```python
from build123d import *

# Parameters (mm, degrees)
SKETCH1_W                = 63.5
SKETCH1_H                = 50.8
BOSS_EXTRUDE1_DEPTH      = 6.35
F_10_32_THREADED_D       = 4.826
F_10_32_THREADED_FRONT_D = 4.826
F_6_32_THREADED_FRONT_D  = 3.5052


with BuildPart() as part:
    # Sketch1 → Boss-Extrude1 (new, symmetric)
    with BuildSketch(Plane.XY):
        with Locations((-31.75, 25.4)):
            Rectangle(SKETCH1_W, SKETCH1_H)
    extrude(amount=BOSS_EXTRUDE1_DEPTH, both=True)

    # #10-32 Threaded (through all)
    with Locations(Plane(origin=(0, 0, 0), x_dir=(0, 0, -1), z_dir=(1, 0, 0))):
        with Locations((0, 44.45), (0, 25.4), (0, 6.35)):
            Hole(F_10_32_THREADED_D / 2)

    # #10-32 Threaded Front (through all)
    with Locations(Plane.XY.offset(6.35)):
        with Locations((-50.8, 38.1), (-25.4, 38.1), (-50.8, 12.7), (-25.4, 12.7)):
            Hole(F_10_32_THREADED_FRONT_D / 2)

    # #6-32 Threaded Front (through all)
    with Locations(Plane.XY.offset(6.35)):
        with Locations((-34.925, 34.925), (-15.875, 34.925), (-15.875, 15.875), (-34.925, 15.875)):
            Hole(F_6_32_THREADED_FRONT_D / 2)


solid = part.part
```
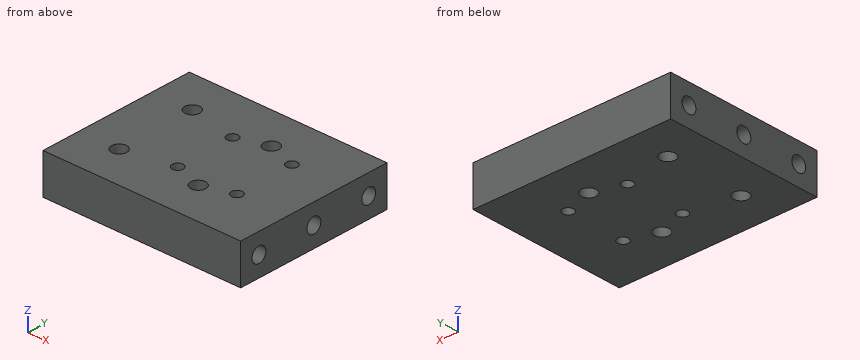
Build history of the part. All positions in model axes, mm. Round coordinates to 2 decimals unless told otherwise and drop trailing zeros. Write each loop counter-clockwise with the first axis right and the second up, starting at its lowest first coordinate (ties: lowest second). Pieces come first, ordered by that corner, then holes.
1) Band-saw the part on D-D, the plane z = -0.5. Give the number of separate pieces and of enclosed holes in the cut face, and give its area (3 significant figures).
2) Band-saw the part on B-B, the plane y = 12.7. List the corners of the cut face in (x, z), and give its area (3 significant figures).
3) Band-saw the part on C-C, the plane y = 6.35. List the corners of the cut face in (x, z), and give its area (3 significant figures).
4) Drill centre lines: probe 1 along Y at (x, z) = (-50.8, -0.25); probe 2 along Y at (x, z) = (-37.5, 0); probe 3 along Z at (x, y) = (-34, 44.5). Where is each one in solid material? Low to high.
5) Band-saw the part on A-A, the plane x = -25.4. List the corners of the cut face in (y, z).
Ans:
1. separate pieces: 4
1. enclosed holes: 8
1. area: 2,210 mm2
2. outline: (-63.5, -6.35) - (-53.21, -6.35) - (-53.21, 6.35) - (-63.5, 6.35) - close; (-48.39, -6.35) - (-27.81, -6.35) - (-27.81, 6.35) - (-48.39, 6.35) - close; (-22.99, -6.35) - (0, -6.35) - (0, 6.35) - (-22.99, 6.35) - close
2. area: 684 mm2
3. outline: (-63.5, -6.35) - (0, -6.35) - (0, -2.41) - (-63.5, -2.41) - close; (-63.5, 2.41) - (0, 2.41) - (0, 6.35) - (-63.5, 6.35) - close
3. area: 500 mm2
4. probe 1: y = 0 to 3.95, 8.75 to 10.29, 15.11 to 23, 27.8 to 35.69, 40.51 to 42.05, 46.85 to 50.8
4. probe 2: y = 0 to 3.94, 8.76 to 22.99, 27.81 to 42.04, 46.86 to 50.8
4. probe 3: z = -6.35 to -2.41, 2.41 to 6.35
5. outline: (0, -6.35) - (10.29, -6.35) - (10.29, 6.35) - (0, 6.35) - close; (15.11, -6.35) - (35.69, -6.35) - (35.69, 6.35) - (15.11, 6.35) - close; (40.51, -6.35) - (50.8, -6.35) - (50.8, 6.35) - (40.51, 6.35) - close; hole circle Ø4.83 at (6.35, 0); hole circle Ø4.83 at (25.4, 0); hole circle Ø4.83 at (44.45, 0)
